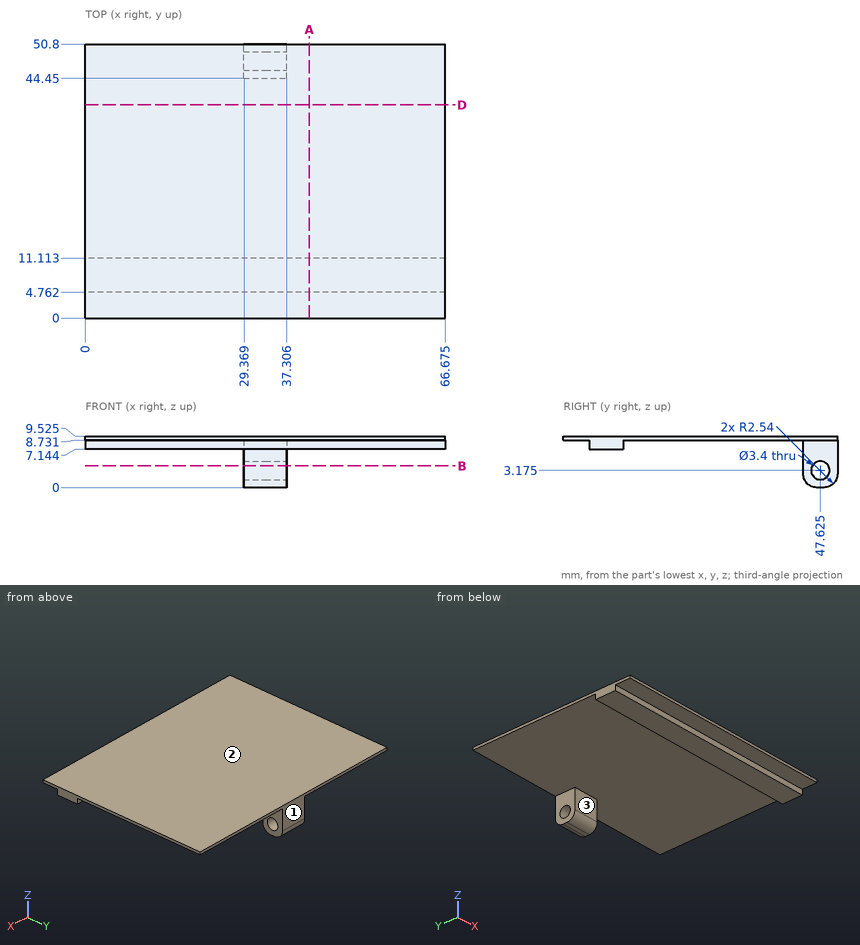
Print and shaded views of the part. All mm, measured from the part's lowest x, y and z. Round coordinates to 2 decimals unless told otherwise and drop trailing zeros. Order: outer loops, then holes, each group sorted by start corner. A loop starts at its lowest first (then second) coordinate and runs counter-clockwise, first axis right, second up.
Q1. Drop flat-ended pins along their axis: pin 1 (10 mm diameter, centred on x = 30, y = 21, fed in from -Z); pin 2 (1.9 mm diameter, centred on x = 19.5, y = 9.5, fed in from -Z); pin 3 (3 mm diameter, centred on y = 46.5, z = 5.5, fed in from +X). Give the stop position or say it passes through.
Q2. Slice it at B-B (z = 4). Write the cut outline in (x, y), and give its area (3 significant figures).
Q3. Two-plate mould, pull along Y, no slides. Class the marked faces 1, 2 and 3: pulls with the +Y half, pulls with the -Y half, needs draft (parallel to the pull), parting line crosses it, or undercut.
Q4. Wall check: L1, parallel to Z at x = 48, y = 32 (1 decimal); L2, parallel to Z at x = 20.5, y = 6.5 (1 decimal); L3, parallel to Y at x = 54.5, z = 8. Give the ranges that are in metal, low to high.
Q5. Slice it at A-A (x = 41.5). Write the cut outline in (y, z) (1 decimal).
Q6. Slice it at D-D (y = 39.5). Write the cut outline in (x, z) (1 decimal).
Results below:
1. pin 1: stops at z = 8.73
1. pin 2: stops at z = 7.14
1. pin 3: stops at x = 37.31
2. outline: (29.37, 44.45) - (37.31, 44.45) - (37.31, 46.14) - (29.37, 46.14) - close; (29.37, 49.11) - (37.31, 49.11) - (37.31, 50.8) - (29.37, 50.8) - close
2. area: 26.8 mm2
3. face 1: pulls with the +Y half
3. face 2: needs draft
3. face 3: undercut
4. L1: z = 8.7 to 9.5
4. L2: z = 7.1 to 9.5
4. L3: y = 4.76 to 11.11
5. outline: (0, 8.7) - (4.8, 8.7) - (4.8, 7.1) - (11.1, 7.1) - (11.1, 8.7) - (50.8, 8.7) - (50.8, 9.5) - (0, 9.5) - close
6. outline: (0, 8.7) - (66.7, 8.7) - (66.7, 9.5) - (0, 9.5) - close
